Input: part model. Units: mm. Frame: model coordinates. A direction names the side the tool comes from. Coordinates: 2 decimals unless noted, no trailing zeros. Loops run counter-clockwise (first coordinate to the right, second up) from the corner with the lowest first, then second, coordinate; pieces in that order, holes last. Notation, with made-up numbers: (0.25, -14.75) - (47.25, -14.75) arc R33 cw to (47.25, 21.25) - close; hole circle Ø3 at (-9.5, -31.75). An arc over 180 degrees is marked (long way). Use one line per item in the form item = value.
from build123d import *

# Parameters (mm, degrees)
EXTRUDE_1_DEPTH     = 14
EXTRUDE_1_DRAFT     = -0.67
CUT_EXTRUDE_1_DEPTH = 7
CUT_EXTRUDE_1_TAPER = 0.67
SKETCH_3_W          = 2
SKETCH_3_H          = 1.5
EXTRUDE_2_DEPTH     = 3


with BuildPart() as part:
    # 草图1 → 凸台-拉伸1 (with draft: the straight prism first)
    with BuildSketch(Plane.XY):
        Polygon((1.876388375, 3.25), (-1.876388375, 3.25), (-3.75277675, 0), (-1.876388375, -3.25), (1.876388375, -3.25), (3.75277675, 0), align=None)
    extrude(amount=EXTRUDE_1_DEPTH)
    # 凸台-拉伸1: the draft: its side faces are tilted about the plane it starts from
    extrude_1_sides = [part.faces().sort_by_distance(p)[0] for p in [
        (0, 3.25, 7),
        (-2.814582562, 1.625, 7),
        (-2.814582562, -1.625, 7),
        (0, -3.25, 7),
        (2.814582562, -1.625, 7),
        (2.814582562, 1.625, 7),
    ]]
    draft(extrude_1_sides, Plane.XY, EXTRUDE_1_DRAFT)

    # 草图2 → 切除-拉伸1 (cut)
    with BuildSketch(Plane.XY.offset(14)):
        with BuildLine():
            Line((1.5, -1.322875656), (1.5, 1.322875656))
            ThreePointArc((1.5, 1.322875656), (-2, 0), (1.5, -1.322875656))
        make_face()
    extrude(amount=-CUT_EXTRUDE_1_DEPTH, taper=CUT_EXTRUDE_1_TAPER, mode=Mode.SUBTRACT)

    # 草图3 → 凸台-拉伸2 (add)
    with BuildSketch(Plane.XY.offset(14)):
        with Locations((0, 2.663719346)):
            Rectangle(SKETCH_3_W, SKETCH_3_H)
        with Locations((0, -2.663719346)):
            Rectangle(SKETCH_3_W, SKETCH_3_H)
    extrude(amount=EXTRUDE_2_DEPTH)


solid = part.part
Q1. Cut plane B-B, the plane y = 2.5. Return loops of the section in (x, z), then the cut area to 3 significant figures.
Check values:
outline = (-2.5, 14) - (-2.31, 0) - (2.31, 0) - (2.5, 14) - (1, 14) - (1, 17) - (-1, 17) - (-1, 14) - close
area = 73.3 mm²
Q2. Set-up query: faces 4 (the flat face through (1, -3, 15)), 5 (the flat face through (0, 1.914, 15)), 6 (the flat face through (0, 0, 0)). Return all of +Z, -Z, +X, -X, +Y, -Y with unobstructed straight access to the full face (end or side cutting, diameter ignored); none if empty.
Check values:
face_4 = +Z, +X, +Y, -Y
face_5 = +Z, +X, -X
face_6 = -Z, +X, -X, +Y, -Y
Q3. First-contact query: P1, Ø1.6, axis at y = -2.5, z = 15, coming from the -X side; P2, Ø1.2, axis at y = -2.5, z = 15.5, coming from the +X side; P3, Ø1, axis at x = -2, y = 0.5, coming from the +Z side. Flat tips, straight axial feed; report the tip coordinate or a pass-through.
Check values:
P1 = -1
P2 = 1
P3 = 14
Q4. Pull-direction query (Y, two-part tool) for faces 1 (the flat face through (0, -1.914, 15)), 2 (the flat face through (0, 3.414, 15)), 3 (the flat face through (-1, 3, 15)); classes: pulls with the +Y half, pulls with the -Y half, needs draft (parallel to the pull), parting line crosses it, or undercut.
Check values:
face_1 = undercut
face_2 = pulls with the +Y half
face_3 = needs draft
Q5. Cut plane A-A, the plane z = 14.5. Return loops of the section in (x, y), then the cut area to 3 significant figures.
Check values:
outline = (-1, -3.41) - (1, -3.41) - (1, -1.91) - (-1, -1.91) - close; (-1, 1.91) - (1, 1.91) - (1, 3.41) - (-1, 3.41) - close
area = 6.00 mm²
Q6. Ray query, line 1 along X through (y, z) = (2, 15.25); line 2 along Z through (x, y) = (-2, 1.5); line 3 along X through (y, z) = (-1, 7.75). Return the intervals inside material, ascending. Write a range as [from, to].
Check values:
line_1 = [-1, 1]
line_2 = [0, 14]
line_3 = [-3.28, -1.65], [1.43, 3.28]
Q7. Cut plane C-C, the plane x = -3. Return loops of the section in (y, z), then the cut area to 3 significant figures.
Check values:
outline = (-1.63, 14) - (-1.3, 0) - (1.3, 0) - (1.63, 14) - close
area = 41.1 mm²
Q8. Cut plane D-D, the plane z = 6. Return loops of the section in (x, y), then the cut area to 3 significant figures.
Check values:
outline = (-3.83, 0) - (-1.92, -3.32) - (1.92, -3.32) - (3.83, 0) - (1.92, 3.32) - (-1.92, 3.32) - close
area = 38.2 mm²
